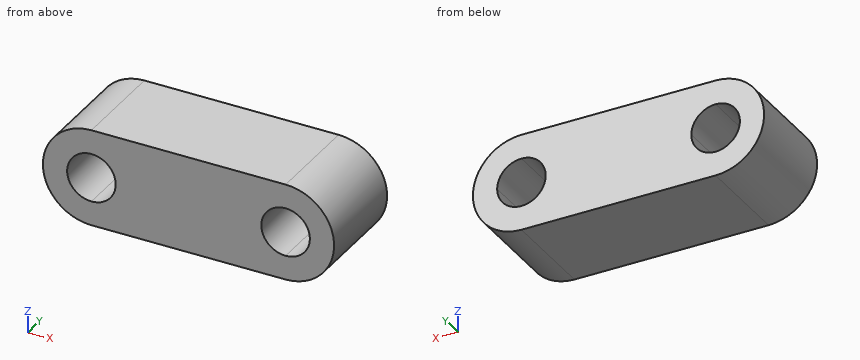
from build123d import *

# Parameters (mm, degrees)
F1_DEPTH = 20


with BuildPart() as f1:
    # F0 (on Front) → F1 (new body)
    with BuildSketch(Plane.XZ):
        with BuildLine():
            Line((0, 5), (0, 0))
            Line((0, 0), (40, 0))
            Line((40, 0), (40, 5))
            ThreePointArc((40, 5), (35, 10), (40, 15))
            Line((40, 15), (40, 20))
            Line((40, 20), (0, 20))
            Line((0, 20), (0, 15))
            ThreePointArc((0, 15), (3.535534, 13.535534), (5, 10))
            ThreePointArc((5, 10), (3.535534, 6.464466), (0, 5))
        make_face()
        with BuildLine():
            ThreePointArc((0, 20), (-10, 10), (0, 0))
            Line((0, 0), (0, 5))
            ThreePointArc((0, 5), (-5, 10), (0, 15))
            Line((0, 15), (0, 20))
        make_face()
        with BuildLine():
            Line((40, 5), (40, 0))
            ThreePointArc((40, 0), (50, 10), (40, 20))
            Line((40, 20), (40, 15))
            ThreePointArc((40, 15), (43.535534, 13.535534), (45, 10))
            ThreePointArc((45, 10), (43.535534, 6.464466), (40, 5))
        make_face()
    extrude(amount=F1_DEPTH)


solid = f1.part
Part model, mm, in its own coordinate system. Round coordinates to 2 decimals unless told otherwise and drop trailing zeros. Order: outer loops, then holes, each group sorted by start corner. A loop starts at its lowest first (then second) coordinate and runs counter-clockwise, first axis right, second up. Notation, with made-up numbers: (-29.75, 16.5) -> (5.25, 16.5) arc R14 cw to (5.25, 41.5) -> close; hole circle Ø2 at (33, 68). An arc over 180 degrees is marked (long way). Put each result on its own line as item: value.
Q1. Wall check: line 1 (X direction, y = -7, z = 9.75); line 2 (X direction, y = -16.5, z = 7.25); line 3 (X direction, y = -17.5, z = 2.75). Give the ranges that are in metal, low to high. Write a range as [from, to].
From the geometry:
line 1: x = [-10, -4.99], [4.99, 35.01], [44.99, 50]
line 2: x = [-9.61, -4.18], [4.18, 35.82], [44.18, 49.61]
line 3: x = [-6.89, 46.89]
Q2. Band-saw the part on A-A (x = 36). Give the cut face in (y, z), and give its area (3 significant figures).
From the geometry:
outline: (-20, 0) -> (0, 0) -> (0, 7) -> (-20, 7) -> close; (-20, 13) -> (0, 13) -> (0, 20) -> (-20, 20) -> close
area: 280 mm2
Q3. Pin check, flat tips, straight feed: pin 1 Ø1 at (y, z) = (-3, 4) entering from -X; pin 2 Ø2 at (y, z) = (-13.5, 3.5) entering from +X; pin 3 Ø8 at (y, z) = (-13.5, 14.5) entering from -X. Stop position of each tip, or through.
From the geometry:
pin 1: stops at x = -8.35
pin 2: stops at x = 48.35
pin 3: stops at x = -9.99
Q4. Band-saw the part on D-D (z = 1.75). Give the cut face in (x, y).
From the geometry:
outline: (-5.65, -20) -> (45.65, -20) -> (45.65, 0) -> (-5.65, 0) -> close
Q5. Band-saw the part on C-C (x = -3). Give the cut face in (y, z), and give its area (3 significant figures).
From the geometry:
outline: (-20, 0.46) -> (0, 0.46) -> (0, 6) -> (-20, 6) -> close; (-20, 14) -> (0, 14) -> (0, 19.54) -> (-20, 19.54) -> close
area: 222 mm2
Q6. Band-saw the part on B-B (y = -1.25). Give the cut face in (x, z).
From the geometry:
outline: (0, 0) -> (40, 0) arc R10 ccw to (40, 20) -> (0, 20) arc R10 ccw to start; hole circle Ø10 at (0, 10); hole circle Ø10 at (40, 10)
